Design review of the part built by this model. Coordinates are the model's own, in mm. Coordinates: 2 decimals unless noted, no trailing zeros. Write each loop counter-clockwise with the first axis right and the second up, starting at its lowest first coordinate (ties: lowest second). Pieces come first, ordered by that corner, then holes.
Q1. Add section D-D, the plane y = 12. Give the boundary of the cut face in (x, z).
Q2. Add section B-B, the plane z = 0.2. Give the number of separate pieces and of enclosed holes in the cut face, plus the area to 3 significant figures.
Q3. Clearance check with a flat-ended pin moving along its axis: pin 1 Ø1.8 at (x, y) = (64.86, 0) entering from -Z. State where the tip first meets the part, or that it passes through.
Q4. To check wall thickness, follow probe 1 along Y at (x, z) = (3.5, -0.6); probe 2 along Y at (x, z) = (68.5, -2.7); probe 3 along X at (y, z) = (3, -2). State the ranges of each line that lie inside material, in increasing order.
Q5. Add section A-A, the plane x = 34. Give the boundary of the cut face in (y, z).
from build123d import *

# Parameters (mm, degrees)
SKETCH1_W           = 180
SKETCH1_H           = 50
BOSS_EXTRUDE1_DEPTH = 3
FILLET1_R           = 15
SKETCH3_R           = 4
SKETCH3_R_2         = 2
CUT_EXTRUDE1_DEPTH  = 8
SKETCH4_R           = 1.5
SKETCH4_W           = 22.5
SKETCH4_H           = 11.9
CUT_EXTRUDE2_DEPTH  = 10


with BuildPart() as part:
    # Sketch1 → Boss-Extrude1 (new body, symmetric)
    with BuildSketch(Plane.XY):
        with Locations((17.559596495, 0)):
            Rectangle(SKETCH1_W, SKETCH1_H)
    extrude(amount=BOSS_EXTRUDE1_DEPTH, both=True)

    # Fillet1
    fillet1_edges = [part.edges().sort_by_distance(p)[0] for p in [
        (107.559596495, -25, 0),
        (-72.440403505, -25, 0),
        (-72.440403505, 25, 0),
        (107.559596495, 25, 0),
    ]]
    fillet(fillet1_edges, radius=FILLET1_R)

    # Sketch3 → Cut-Extrude1 (cut)
    with BuildSketch(Plane.XY.offset(3)):
        with Locations((-47.926163707, 0)):
            Circle(SKETCH3_R)
        with Locations((-47.926163707, 12)):
            Circle(SKETCH3_R_2)
        with Locations((-47.926163707, -12)):
            Circle(SKETCH3_R_2)
        with Locations((-59.926163707, 0)):
            Circle(SKETCH3_R_2)
        with Locations((-35.926163707, 0)):
            Circle(SKETCH3_R_2)
    extrude(amount=-CUT_EXTRUDE1_DEPTH, mode=Mode.SUBTRACT)

    # Sketch4 → Cut-Extrude2 (cut)
    with BuildSketch(Plane.XY.offset(3)):
        with Locations((64.859596495, 0)):
            Circle(SKETCH4_R)
        with Locations((91.759596495, 0)):
            Circle(SKETCH4_R)
        with Locations((78.309596495, 0)):
            Rectangle(SKETCH4_W, SKETCH4_H)
        with BuildLine():
            Line((-9.269868987, 8.287867606), (40.115980257, 8.287867606))
            ThreePointArc((40.115980257, 8.287867606), (48.403847863, 0), (40.115980257, -8.287867606))
            Line((40.115980257, -8.287867606), (-9.269868987, -8.287867606))
            ThreePointArc((-9.269868987, -8.287867606), (-17.557736593, 0), (-9.269868987, 8.287867606))
        make_face()
    extrude(amount=-CUT_EXTRUDE2_DEPTH, mode=Mode.SUBTRACT)


solid = part.part
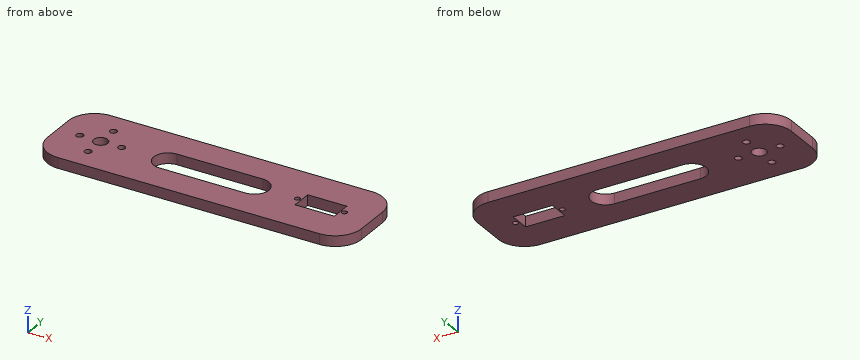
Here are the results:
1. outline: (-72.31, -3) - (-49.93, -3) - (-49.93, 3) - (-72.31, 3) - close; (-45.93, -3) - (107.43, -3) - (107.43, 3) - (-45.93, 3) - close
2. separate pieces: 1
2. enclosed holes: 9
2. area: 7,390 mm2
3. pin 1: passes through
4. probe 1: y = -25 to -8.29, 8.29 to 25
4. probe 2: y = -25 to -5.95, 5.95 to 25
4. probe 3: x = -72.44 to -50.57, -45.28 to -17, 47.84 to 67.06, 89.56 to 107.56
5. outline: (-25, -3) - (-8.29, -3) - (-8.29, 3) - (-25, 3) - close; (8.29, -3) - (25, -3) - (25, 3) - (8.29, 3) - close
